Geometry check sheet. Reference: the model listing, model coordinates, mm. A direction names the side the tool comes from. Give positions to 0.01 mm unless a question says otherwise; leave off trailing zeros. Write each loop counter-clockwise with the first axis right and the second up, starting at its lowest first coordinate (ties: lowest second). Pieces come first, ordered by that corner, then holes. Notation, with made-up numbers: (-37.75, 6) -> (9.25, 6) arc R11 ccw to (9.25, 23) -> close; hole circle Ø8 at (57.5, 66.5). An arc over 180 degrees is marked (long way). Write item = value, one per line. Start each with the question number.
1. Set-up check for faces 1 (the flat face through (3, 22, 6.35)), 2 (the flat face through (3, 6.35, 92)), 3 (the flat face through (3, 12.7, 3)), 4 (the flat face through (3, 95.25, 124)), 5 (the flat face through (3, 124, 114.3)): record each of +Z, -Z, +X, -X, +Y, -Y from which the full face is reachable in a straight line by a thin tool's end or side.
2. Depth check by flat-ended pin: P1, Ø1.9, axis at x = 2, z = 66, coming from the -Y side; P2, Ø3, axis at x = 4.5, y = 125.5, coming from the +Z side; P3, Ø3, axis at x = 3, y = 125, coming from the -Z side. Enter the tip coordinate at first touch or a pass-through.
3. Cross-section at A-A, the plane y = 46.5. Record the cut outline in (x, z).
4. Thickness scan on line 1 along Z through (x, y) = (4.25, 9.5); line 2 along Y through (x, z) = (2.25, 72.5). Record the ranges inside material, lowest first.
```python
from build123d import *

# Parameters (mm, degrees)
F1_DEPTH = 6.35


# Not quite as in the source:
# - a feature names something its author has since deleted; it is built from what else it names


with BuildPart() as f1:
    # F0 (on Right) → F1 (new body)
    with BuildSketch(Plane.YZ):
        Polygon((12.7, 127), (6.35, 127), (0, 127), (0, 120.65), (6.35, 120.65), (6.35, 114.3), (0, 114.3), (0, 107.95), (6.35, 107.95), (6.35, 101.6), (0, 101.6), (0, 95.25), (6.35, 95.25), (6.35, 88.9), (0, 88.9), (0, 82.55), (6.35, 82.55), (6.35, 76.2), (0, 76.2), (0, 69.85), (6.35, 69.85), (6.35, 63.5), (0, 63.5), (0, 57.15), (6.35, 57.15), (6.35, 50.8), (0, 50.8), (0, 44.45), (6.35, 44.45), (6.35, 38.1), (0, 38.1), (0, 31.75), (6.35, 31.75), (6.35, 25.4), (0, 25.4), (0, 19.05), (6.35, 19.05), (6.35, 12.7), (0, 12.7), (0, 6.35), (6.35, 6.35), (12.7, 6.35), (12.7, 0), (19.05, 0), (19.05, 6.35), (25.4, 6.35), (25.4, 0), (31.75, 0), (31.75, 6.35), (38.1, 6.35), (38.1, 0), (44.45, 0), (44.45, 6.35), (50.8, 6.35), (50.8, 0), (57.15, 0), (57.15, 6.35), (63.5, 6.35), (63.5, 0), (69.85, 0), (69.85, 6.35), (76.2, 6.35), (76.2, 0), (82.55, 0), (82.55, 6.35), (88.9, 6.35), (88.9, 0), (95.25, 0), (95.25, 6.35), (101.6, 6.35), (101.6, 0), (107.95, 0), (107.95, 6.35), (114.3, 6.35), (114.3, 0), (120.65, 0), (120.65, 6.35), (120.65, 12.7), (127, 12.7), (127, 19.05), (120.65, 19.05), (120.65, 25.4), (127, 25.4), (127, 31.75), (120.65, 31.75), (120.65, 38.1), (127, 38.1), (127, 44.45), (120.65, 44.45), (120.65, 50.8), (127, 50.8), (127, 57.15), (120.65, 57.15), (120.65, 63.5), (127, 63.5), (127, 69.85), (120.65, 69.85), (120.65, 76.2), (127, 76.2), (127, 82.55), (120.65, 82.55), (120.65, 88.9), (127, 88.9), (127, 95.25), (120.65, 95.25), (120.65, 101.6), (127, 101.6), (127, 107.95), (120.65, 107.95), (120.65, 114.3), (127, 114.3), (127, 120.65), (120.65, 120.65), (114.3, 120.65), (114.3, 127), (107.95, 127), (107.95, 120.65), (101.6, 120.65), (101.6, 127), (95.25, 127), (95.25, 120.65), (88.9, 120.65), (88.9, 127), (82.55, 127), (82.55, 120.65), (76.2, 120.65), (76.2, 127), (69.85, 127), (69.85, 120.65), (63.5, 120.65), (63.5, 127), (57.15, 127), (57.15, 120.65), (50.8, 120.65), (50.8, 127), (44.45, 127), (44.45, 120.65), (38.1, 120.65), (38.1, 127), (31.75, 127), (31.75, 120.65), (25.4, 120.65), (25.4, 127), (19.05, 127), (19.05, 120.65), (12.7, 120.65), align=None)
    extrude(amount=F1_DEPTH)


solid = f1.part
```
Answers:
q1.face_1 = -Z, +X, -X
q1.face_2 = +X, -X, -Y
q1.face_3 = -Z, +X, -X, -Y
q1.face_4 = +Z, +X, -X
q1.face_5 = +X, -X, +Y
q2.P1 = 6.35
q2.P2 = 120.65
q2.P3 = 12.7
q3.outline = (0, 6.35) -> (6.35, 6.35) -> (6.35, 127) -> (0, 127) -> close
q4.line_1 = 6.35 to 127
q4.line_2 = 0 to 120.65
